from build123d import *

# Parameters (mm, degrees)
F1_DEPTH = 12.7
F2_DEPTH = 95.25


# Not quite as in the source:
# - a feature names something its author has since deleted; it is built from what else it names


with BuildPart() as f1:
    # F0 (on Front) → F1 (new body)
    with BuildSketch(Plane.XZ):
        Polygon((-187.5869779497, -91.9575006988), (-169.2561069029, -60.2075006988), (-187.5869779497, -28.4575006988), (-224.2487200432, -28.4575006988), (-242.57959109, -60.2075006988), (-224.2487200432, -91.9575006988), align=None)
        Polygon((-222.4156329385, -88.7825006988), (-238.9134168806, -60.2075006988), (-222.4156329385, -31.6325006988), (-189.4200650544, -31.6325006988), (-172.9222811123, -60.2075006988), (-189.4200650544, -88.7825006988), align=None, mode=Mode.SUBTRACT)
        Polygon((-59.2708806223, -60.2075006988), (-77.6017516691, -28.4575006988), (-114.2634937626, -28.4575006988), (-132.5943648094, -60.2075006988), (-114.2634937626, -91.9575006988), (-77.6017516691, -91.9575006988), align=None)
        Polygon((-112.4304066579, -88.7825006988), (-128.9281906, -60.2075006988), (-112.4304066579, -31.6325006988), (-79.4348387737, -31.6325006988), (-62.9370548316, -60.2075006988), (-79.4348387737, -88.7825006988), align=None, mode=Mode.SUBTRACT)
        Polygon((-77.6017516691, -28.4575006988), (-59.2708806223, 3.2924993012), (-77.6017516691, 35.0424993012), (-114.2634937626, 35.0424993012), (-132.5943648094, 3.2924993012), (-114.2634937626, -28.4575006988), align=None)
        Polygon((-112.4304066579, -25.2825006988), (-128.9281906, 3.2924993012), (-112.4304066579, 31.8674993012), (-79.4348387737, 31.8674993012), (-62.9370548316, 3.2924993012), (-79.4348387737, -25.2825006988), align=None, mode=Mode.SUBTRACT)
        Polygon((-132.5943648094, -60.2075006988), (-114.2634937626, -28.4575006988), (-132.5943648094, 3.2924993012), (-169.2561069029, 3.2924993012), (-187.5869779497, -28.4575006988), (-169.2561069029, -60.2075006988), align=None)
        Polygon((-167.4230197982, -57.0325006988), (-183.9208037403, -28.4575006988), (-167.4230197982, 0.1174993012), (-134.4274519141, 0.1174993012), (-117.929667972, -28.4575006988), (-134.4274519141, -57.0325006988), align=None, mode=Mode.SUBTRACT)
        Polygon((-222.4156329385, -31.6325006988), (-238.9134168806, -60.2075006988), (-222.4156329385, -88.7825006988), (-189.4200650544, -88.7825006988), (-172.9222811123, -60.2075006988), (-189.4200650544, -31.6325006988), align=None)
        Polygon((-112.4304066579, -31.6325006988), (-128.9281906, -60.2075006988), (-112.4304066579, -88.7825006988), (-79.4348387737, -88.7825006988), (-62.9370548316, -60.2075006988), (-79.4348387737, -31.6325006988), align=None)
        Polygon((-167.4230197982, 0.1174993012), (-183.9208037403, -28.4575006988), (-167.4230197982, -57.0325006988), (-134.4274519141, -57.0325006988), (-117.929667972, -28.4575006988), (-134.4274519141, 0.1174993012), align=None)
        Polygon((-112.4304066579, 31.8674993012), (-128.9281906, 3.2924993012), (-112.4304066579, -25.2825006988), (-79.4348387737, -25.2825006988), (-62.9370548316, 3.2924993012), (-79.4348387737, 31.8674993012), align=None)
    extrude(amount=F1_DEPTH)

    # F0 (on Front) → F2 (join)
    with BuildSketch(Plane.XZ):
        Polygon((-77.6017516691, -28.4575006988), (-59.2708806223, 3.2924993012), (-77.6017516691, 35.0424993012), (-114.2634937626, 35.0424993012), (-132.5943648094, 3.2924993012), (-114.2634937626, -28.4575006988), align=None)
        Polygon((-112.4304066579, -25.2825006988), (-128.9281906, 3.2924993012), (-112.4304066579, 31.8674993012), (-79.4348387737, 31.8674993012), (-62.9370548316, 3.2924993012), (-79.4348387737, -25.2825006988), align=None, mode=Mode.SUBTRACT)
        Polygon((-59.2708806223, -60.2075006988), (-77.6017516691, -28.4575006988), (-114.2634937626, -28.4575006988), (-132.5943648094, -60.2075006988), (-114.2634937626, -91.9575006988), (-77.6017516691, -91.9575006988), align=None)
        Polygon((-112.4304066579, -88.7825006988), (-128.9281906, -60.2075006988), (-112.4304066579, -31.6325006988), (-79.4348387737, -31.6325006988), (-62.9370548316, -60.2075006988), (-79.4348387737, -88.7825006988), align=None, mode=Mode.SUBTRACT)
        Polygon((-132.5943648094, -60.2075006988), (-114.2634937626, -28.4575006988), (-132.5943648094, 3.2924993012), (-169.2561069029, 3.2924993012), (-187.5869779497, -28.4575006988), (-169.2561069029, -60.2075006988), align=None)
        Polygon((-167.4230197982, -57.0325006988), (-183.9208037403, -28.4575006988), (-167.4230197982, 0.1174993012), (-134.4274519141, 0.1174993012), (-117.929667972, -28.4575006988), (-134.4274519141, -57.0325006988), align=None, mode=Mode.SUBTRACT)
        Polygon((-187.5869779497, -91.9575006988), (-169.2561069029, -60.2075006988), (-187.5869779497, -28.4575006988), (-224.2487200432, -28.4575006988), (-242.57959109, -60.2075006988), (-224.2487200432, -91.9575006988), align=None)
        Polygon((-222.4156329385, -88.7825006988), (-238.9134168806, -60.2075006988), (-222.4156329385, -31.6325006988), (-189.4200650544, -31.6325006988), (-172.9222811123, -60.2075006988), (-189.4200650544, -88.7825006988), align=None, mode=Mode.SUBTRACT)
        Polygon((-57.4378374826, -63.3825006988), (-59.2708806223, -60.2075006988), (-77.6017516691, -91.9575006988), (-114.2634937626, -91.9575006988), (-132.5943648094, -60.2075006988), (-169.2561069029, -60.2075006988), (-187.5869779497, -91.9575006988), (-224.2487200432, -91.9575006988), (-242.57959109, -60.2075006988), (-224.2487200432, -28.4575006988), (-187.5869779497, -28.4575006988), (-169.2561069029, 3.2924993012), (-172.9222811123, 3.2924993012), (-189.4200540638, -25.2824816625), (-226.0817961573, -25.2824816625), (-246.24577629, -60.2075197352), (-226.0817961573, -95.1325578078), (-185.7539677819, -95.1325578078), (-167.4230967351, -63.3825578078), (-134.4273749772, -63.3825578078), (-116.0965039304, -95.1325578078), (-75.7687415012, -95.1325578078), align=None)
    extrude(amount=F2_DEPTH)


solid = f1.part
Check sheet for the modelled part. Datum: model origin and axes. Units: mm. A direction names the side the tool comes from. Coordinates: 2 decimals unless noted, no trailing zeros. Write each loop counter-clockwise with the first axis right and the second up, starting at its lowest first coordinate (ties: lowest second). Pieces come first, ordered by that corner, then holes. Notation, with made-up numbers: M -0.75,86 L 42.25,86 A28 ccw 42.25,119 Z; hole C 16.25,27.5 d10. An arc over 180 degrees is marked long. Answer as CSV lines item,"result".
Q1. Material ranges on probe 1 along X at (y, z) = (-59, -9.5); probe 2 along Z at (x, y) = (-126, -38.5); probe 3 along X at (y, z) = (-78, -36.5), recorded low to high. Write a range as from..to.
Check result:
probe 1,"-180.31..-172.98, -128.87..-121.54, -70.32..-66.66"
probe 2,"-77.98..-65.28, -55.14..-42.44, -14.48..-1.78, 8.36..14.71"
probe 3,"-232.56..-225.23, -186.61..-179.28, -122.57..-115.24, -76.62..-72.96"
Q2. Cross-section at B-B (x = -73.5). Record the boundary of the cut face in (y, z), then the cut area to 3 significant figures.
Check result:
outline,"M -95.25,-91.2 L 0,-91.2 L 0,-35.56 L -95.25,-35.56 L -95.25,-41.91 L -12.7,-41.91 L -12.7,-78.5 L -95.25,-78.5 Z; M -95.25,-21.35 L 0,-21.35 L 0,27.94 L -95.25,27.94 L -95.25,21.59 L -12.7,21.59 L -12.7,-15 L -95.25,-15 Z"
area,"3,950 mm^2"
Q3. Set-up check for faces 1 (the face through (-71.07, -53.397, -10.795)), 2 (the face through (-236.305, -46.958, -77.426)), 3 (the face through (-176.717, -46.958, -79.48)): record each of +Z, -Z, +X, -X, +Y, -Y from which the full face is reachable in a straight line by a thin tool's end or side.
Check result:
face 1,"-Y"
face 2,"-Z, -X, +Y, -Y"
face 3,"-Z, +Y, -Y"
Q4. Cross-section at C-C (x = -160). Record the boundary of the cut face in (y, z).
Check result:
outline,"M -95.25,-63.38 L 0,-63.38 L 0,3.29 L -95.25,3.29 L -95.25,0.12 L -12.7,0.12 L -12.7,-57.03 L -95.25,-57.03 Z"
Q5. Go/stop test with flat-tipped pins: pin 1 (10 mm diameter, centred on x = -153.5, y = -55.5, fed in from -Z); pin 2 (3 mm diameter, centred on y = -54, z = 11, fed in from -X); pin 3 (3 mm diameter, centred on y = -59.5, z = -19, fed in from +X). Record where each tip stops, or that it passes through.
Check result:
pin 1,"z = -63.38"
pin 2,"x = -129.01"
pin 3,"x = -71.28"
Q6. Mould release check, pull along X, two halves, no side actions. Record for faces 4 (the face through (-96, -47, -95.133)), 5 (the face through (-123.3, -46.96, 19.39)), 6 (the face through (-206, -53, -88.783)), 7 (the face through (-96, -53, -31.633)): released by +X, released by -X, zero draft, split by the parting line, or undercut.
Check result:
face 4,"zero draft"
face 5,"released by -X"
face 6,"undercut"
face 7,"undercut"
Q7. Cross-section at A-A (z = -83). Record the boundary of the cut face in (x, y).
Check result:
outline,"M -233.09,-95.25 L -225.75,-95.25 L -225.75,-12.7 L -186.08,-12.7 L -186.08,-95.25 L -178.75,-95.25 L -178.75,0 L -233.09,0 Z; M -123.1,-95.25 L -115.77,-95.25 L -115.77,-12.7 L -76.1,-12.7 L -76.1,-95.25 L -68.76,-95.25 L -68.76,0 L -123.1,0 Z"
Q8. Cross-section at D-D (y = -51). Count the separate pieces of the cut face and the enclosed holes in it, then the cut area to 3 significant figures.
Check result:
separate pieces,"1"
enclosed holes,"4"
area,"3,830 mm^2"
